```python
from build123d import *


with BuildPart() as f1:
    # F0 (on Front) → F1 (revolve)
    with BuildSketch(Plane.XZ):
        with BuildLine():
            ThreePointArc((10.1356245577, 37.6246646047), (13.3272956222, 45.1520650335), (14.128446579, 53.2888136804))
            ThreePointArc((14.128446579, 53.2888136804), (12.2078947119, 55.5624464713), (10.1356245577, 57.6987100202))
            Line((10.1356245577, 57.6987100202), (4.9142432399, 51.845254764))
            Line((4.9142432399, 51.845254764), (7.6890488201, 59.8808432291))
            ThreePointArc((7.6890488201, 59.8808432291), (3.9800972298, 62.6257206248), (0, 64.9601370096))
            Line((0, 64.9601370096), (0, 0))
            Line((0, 0), (16.2784270942, 0))
            Line((16.2784270942, 0), (16.2784270942, 9.6749141812))
            Line((16.2784270942, 9.6749141812), (10.1356245577, 15.5105758458))
            ThreePointArc((10.1356245577, 15.5105758458), (7.6325309522, 26.5676202253), (10.1356245577, 37.6246646047))
        make_face()
    revolve(axis=Axis((0, 0, 32.4800685048), (0, 0, 1)))


solid = f1.part
```
Geometry: final body of the model. Coordinates: model frame, mm. Coordinates: 2 decimals unless noted, no trailing zeros. Order: outer loops, then holes, each group sorted by start corner. A loop starts at its lowest first (then second) coordinate and runs counter-clockwise, first axis right, second up. Notation, with made-up numbers: (-8.5, 66) -> (2.5, 66) arc R34 ccw to (2.5, 101) -> close; hole circle Ø10 at (-18, 32). An arc over 180 degrees is marked (long way). Write each question's results on one line, items separated by ' | '. Start each with the question number.
1) First-contact query: pin 1 (5 mm diameter, centred on y = -4, z = 45, fed in from -X); pin 2 (12 mm diameter, centred on x = 6.5, y = -7.5, fed in from +Z); pin 3 (3 mm diameter, centred on x = 0, z = 53, fed in from -Y). Flat tips, straight axial feed; report the tip coordinate or a pass-through.
2) Material intervals for line 1 along X through (y, z) = (-2, 56); line 2 along Y through (x, z) = (5, 57); line 3 along Y through (x, z) = (11, 53.5), sorted ascending.
3) Cut plane A-A, the plane z = 18. Output: boundary loops of the cut face in (x, y), and give its area (3 significant figures).
4) Mould query, pull axis Z, two halves, no side actions, for faces 1 (the conical face through (-8.28, -6.349, 15.227)), 2 (the flat face through (0, 0, 0)), 3 (the cylindrical face through (-3.53, -15.89, 4.91)). Classes: released by +Z, released by -Z, zero draft, split by the parting line, or undercut.
Checks:
1) pin 1: x = -13.5 | pin 2: z = 62.66 | pin 3: y = -14.17
2) line 1: -11.64 to -8.39, -6.03 to 6.03, 8.39 to 11.64 | line 2: -9.62 to -8.09, -4.45 to 4.45, 8.09 to 9.62 | line 3: -8.6 to 8.6
3) outline: circle Ø18.21 at (0, 0) | area: 260 mm^2
4) face 1: undercut | face 2: released by -Z | face 3: zero draft
